```python
from build123d import *

# Parameters (mm, degrees)
SKETCH1_W               = 39.1
SKETCH1_H               = 33
SKETCH1_R               = 0.95
SKETCH1_R_2             = 4.5
SKETCH1_W_2             = 12.2
SKETCH1_H_2             = 22.7
BOSS_EXTRUDE1_DEPTH     = 4
BOSS_EXTRUDE2_START     = 4
SKETCH2_R               = 8
SKETCH2_R_2             = 4.403773093
BOSS_EXTRUDE2_DEPTH     = 4
CUT_EXTRUDE1_START      = 8
SKETCH3_R               = 5.6
CUT_EXTRUDE1_DEPTH      = 5
SKETCH5_W               = 39.1
SKETCH5_H               = 10
SKETCH5_W_2             = 6.003695208
SKETCH5_H_2             = 43
BOSS_EXTRUDE3_DEPTH     = 4
SKETCH4_R               = 1.65
CUT_EXTRUDE3_DEPTH      = 9
CUT_EXTRUDE3_DEPTH_BACK = 10
CUT_EXTRUDE4_START      = 4
SKETCH6_R               = 3
CUT_EXTRUDE4_DEPTH      = 10
SKETCH7_W               = 6
SKETCH7_H               = 43
BOSS_EXTRUDE4_DEPTH     = 4
SKETCH8_R               = 1.6
CUT_EXTRUDE6_DEPTH      = 4


with BuildPart() as part:
    # Sketch1 → Boss-Extrude1 (new body)
    with BuildSketch(Plane.XY):
        with Locations((-10.45, -5.15)):
            Rectangle(SKETCH1_W, SKETCH1_H)
        with Locations((0, 8.9)):
            Circle(SKETCH1_R, mode=Mode.SUBTRACT)
        with Locations((0, -19.2)):
            Circle(SKETCH1_R, mode=Mode.SUBTRACT)
        with Locations((-20, 0)):
            Circle(SKETCH1_R_2, mode=Mode.SUBTRACT)
        with Locations((0, -5.15)):
            Rectangle(SKETCH1_W_2, SKETCH1_H_2, mode=Mode.SUBTRACT)
    extrude(amount=BOSS_EXTRUDE1_DEPTH)

    # Sketch2 → Boss-Extrude2 (add)
    with BuildSketch(Plane.XY.offset(BOSS_EXTRUDE2_START)):
        with Locations((-20, 0)):
            Circle(SKETCH2_R)
        with Locations((-20, 0)):
            Circle(SKETCH2_R_2, mode=Mode.SUBTRACT)
    extrude(amount=BOSS_EXTRUDE2_DEPTH)

    # Sketch3 → Cut-Extrude1 (cut)
    with BuildSketch(Plane.XY.offset(CUT_EXTRUDE1_START)):
        with Locations((-20, 0)):
            Circle(SKETCH3_R)
    extrude(amount=-CUT_EXTRUDE1_DEPTH, mode=Mode.SUBTRACT)

    # Sketch5 → Boss-Extrude3 (add)
    with BuildSketch(Plane.XY):
        with Locations((-10.45, 16.35)):
            Rectangle(SKETCH5_W, SKETCH5_H)
        with Locations((-33.001847604, -0.15)):
            Rectangle(SKETCH5_W_2, SKETCH5_H_2)
    extrude(amount=BOSS_EXTRUDE3_DEPTH)

    # Sketch4 → Cut-Extrude3 (cut, two sides)
    with BuildSketch(Plane.XY) as cut_extrude3_sk:
        with Locations((-10.5, 16.454482672)):
            Circle(SKETCH4_R)
        with Locations((-29.5, 16.454482672)):
            Circle(SKETCH4_R)
        with Locations((-29.5, -16.454482672)):
            Circle(SKETCH4_R)
        with Locations((-10.5, -16.454482672)):
            Circle(SKETCH4_R)
    extrude(amount=CUT_EXTRUDE3_DEPTH, mode=Mode.SUBTRACT)
    extrude(cut_extrude3_sk.sketch, amount=-CUT_EXTRUDE3_DEPTH_BACK, mode=Mode.SUBTRACT)

    # Sketch6 → Cut-Extrude4 (cut)
    with BuildSketch(Plane.XY.offset(CUT_EXTRUDE4_START)):
        with Locations((-11.9, 8)):
            Circle(SKETCH6_R)
        with Locations((-28.1, 8)):
            Circle(SKETCH6_R)
        with Locations((-11.9, -8)):
            Circle(SKETCH6_R)
        with Locations((-28.1, -8)):
            Circle(SKETCH6_R)
    extrude(amount=-CUT_EXTRUDE4_DEPTH, mode=Mode.SUBTRACT)

    # Sketch7 → Boss-Extrude4 (add)
    with BuildSketch(Plane.XY):
        Polygon((9.1, -21.65), (-36.003695208, -21.65), (-36.003695208, -30.65), (15.1, -30.65), (15.1, -21.65), align=None)
        with Locations((12.1, -0.15)):
            Rectangle(SKETCH7_W, SKETCH7_H)
        Polygon((-36.003695208, 21.35), (9.1, 21.35), (15.1, 21.35), (15.1, 51.35), (-36.003695208, 51.35), align=None)
    extrude(amount=BOSS_EXTRUDE4_DEPTH)

    # Sketch8 → Cut-Extrude6 (cut)
    with BuildSketch(Plane.XY):
        with Locations((9.1, -24.65)):
            Circle(SKETCH8_R)
        with Locations((-30.003695208, -24.65)):
            Circle(SKETCH8_R)
        with Locations((9.1, 45.35)):
            Circle(SKETCH8_R)
    extrude(amount=CUT_EXTRUDE6_DEPTH, mode=Mode.SUBTRACT)


solid = part.part
```
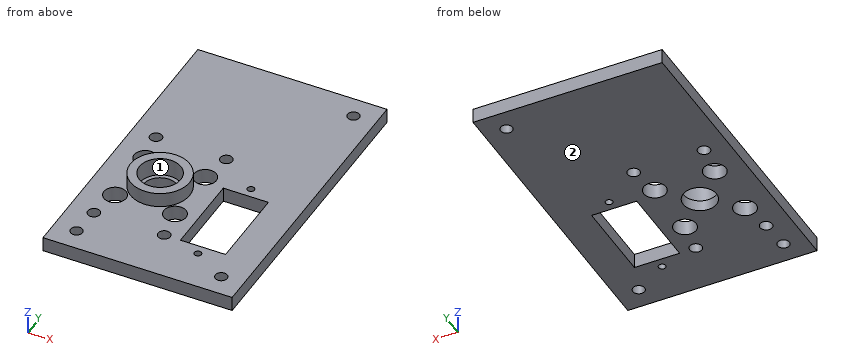
Input: part model. Units: mm. Frame: model coordinates. Face numbers are marked on the shaded views. Give positions to 0.01 mm unless a question says otherwise; leave off trailing zeros. Order: outer loops, then holes, each group sorted by start corner. A loop starts at its lowest first (then second) coordinate and runs counter-clockwise, first axis right, second up. Notation, with made-up numbers: (75.25, 13) -> (116.25, 13) arc R28 cw to (116.25, 47) -> close; hole circle Ø5 at (69.5, 88). An arc over 180 degrees is marked (long way). Write each question's results on one line, items separated by ' | '. Start each with the question number.
Item 1: Mould query, pull axis Y, two halves, no side actions, for the marked faces 1 and 2. Classes: pulls with the +Y half, pulls with the -Y half, needs draft (parallel to the pull), parting line crosses it, or undercut.
Item 2: Line query: line 1 (Y direction, x = 2, z = 2); line 2 (Y direction, x = -10.5, z = 1.1); line 3 (Y direction, x = -20, z = 2.2). Output: solid intervals per line, ascending.
Item 3: Cut plane C-C on y = 0. Return the cut outline in (x, z), then the cut area to 3 significant figures.
Item 4: Cut plane A-A on y = -19.2. Return the cut outline in (x, z), then the cut area to 3 significant figures.
Item 5: Cut plane B-B on x = -30. Return the cut outline in (y, z).
Item 6: Contact query for flat-ended pins moving along their axis: P1, Ø7, axis at x = -20, y = 0, coming from the -Z side; P2, Ø5.5, axis at x = -10.5, y = -16.45, coming from the +Z side; P3, Ø3.5, axis at x = -18, y = 2, coming from the +Z side. Output: stop coordinate, or through.
Item 7: Cut plane D-D on z = 6.25. Return the cut outline in (x, y).
Established:
1) face 1: undercut | face 2: needs draft
2) line 1: -30.65 to -16.5, 6.2 to 51.35 | line 2: -30.65 to -18.1, -14.8 to -10.65, -5.35 to 5.35, 10.65 to 14.8, 18.1 to 51.35 | line 3: -30.65 to -4.5, 4.5 to 51.35
3) outline: (-36, 0) -> (-24.5, 0) -> (-24.5, 3) -> (-25.6, 3) -> (-25.6, 8) -> (-28, 8) -> (-28, 4) -> (-36, 4) -> close; (-15.5, 0) -> (-6.1, 0) -> (-6.1, 4) -> (-12, 4) -> (-12, 8) -> (-14.4, 8) -> (-14.4, 3) -> (-15.5, 3) -> close; (6.1, 0) -> (15.1, 0) -> (15.1, 4) -> (6.1, 4) -> close | area: 137 mm^2
4) outline: (-36, 0) -> (-0.95, 0) -> (-0.95, 4) -> (-36, 4) -> close; (0.95, 0) -> (15.1, 0) -> (15.1, 4) -> (0.95, 4) -> close | area: 197 mm^2
5) outline: (-30.65, 0) -> (-26.25, 0) -> (-26.25, 4) -> (-30.65, 4) -> close; (-23.05, 0) -> (-18.03, 0) -> (-18.03, 4) -> (-23.05, 4) -> close; (-14.88, 0) -> (-10.32, 0) -> (-10.32, 4) -> (-14.88, 4) -> close; (-5.68, 0) -> (5.68, 0) -> (5.68, 4) -> (-5.68, 4) -> close; (10.32, 0) -> (14.88, 0) -> (14.88, 4) -> (10.32, 4) -> close; (18.03, 0) -> (51.35, 0) -> (51.35, 4) -> (18.03, 4) -> close
6) P1: through | P2: z = 4 | P3: z = 3
7) outline: circle Ø16 at (-20, 0); hole circle Ø11.2 at (-20, 0)
